from build123d import *

# Parameters (mm, degrees)
CYLINDER001_R     = 1.5
CYLINDER001_DEPTH = 40
CYLINDER_R        = 1.5
CYLINDER_DEPTH    = 40
BOX003_W          = 10
BOX003_H          = 40
BOX003_DEPTH      = 25
BOX002_W          = 5
BOX002_H          = 35
BOX002_DEPTH      = 35
BOX001_W          = 10
BOX001_H          = 40
BOX001_DEPTH      = 25
BOX_W             = 35
BOX_H             = 40
BOX_DEPTH         = 35
FILLET_R          = 10


with BuildPart() as cylinder001:
    # Cylinder001 → Cylinder001 (new body)
    with BuildSketch(Plane(origin=(27.5, 20, 0), x_dir=(1, 0, 0), z_dir=(0, 0, 1))):
        Circle(CYLINDER001_R)
    extrude(amount=CYLINDER001_DEPTH)


with BuildPart() as cylinder:
    # Cylinder → Cylinder (new body)
    with BuildSketch(Plane(origin=(12.5, 20, 0), x_dir=(1, 0, 0), z_dir=(0, 0, 1))):
        Circle(CYLINDER_R)
    extrude(amount=CYLINDER_DEPTH)


with BuildPart() as cube003:
    # Box003 → Box003 (new body)
    with BuildSketch(Plane(origin=(25, 0, 10), x_dir=(1, 0, 0), z_dir=(0, 0, 1))):
        with Locations((5, 20)):
            Rectangle(BOX003_W, BOX003_H)
    extrude(amount=BOX003_DEPTH)


with BuildPart() as cube002:
    # Box002 → Box002 (new body)
    with BuildSketch(Plane(origin=(15, 0, 5), x_dir=(1, 0, 0), z_dir=(0, 0, 1))):
        with Locations((2.5, 17.5)):
            Rectangle(BOX002_W, BOX002_H)
    extrude(amount=BOX002_DEPTH)


with BuildPart() as cube001:
    # Box001 → Box001 (new body)
    with BuildSketch(Plane.XY.offset(10)):
        with Locations((5, 20)):
            Rectangle(BOX001_W, BOX001_H)
    extrude(amount=BOX001_DEPTH)


with BuildPart() as cut004:
    # Box → Box (new body)
    with BuildSketch(Plane.XY):
        with Locations((17.5, 20)):
            Rectangle(BOX_W, BOX_H)
    extrude(amount=BOX_DEPTH)

    # Fillet
    fillet_edges = [cut004.edges().sort_by_distance(p)[0] for p in [
        (0, 0, 17.5),
        (0, 40, 17.5),
        (35, 0, 17.5),
        (35, 40, 17.5),
        (17.5, 0, 35),
        (17.5, 40, 35),
    ]]
    fillet(fillet_edges, radius=FILLET_R)

    # Cut: cut Cube001
    add(cube001.part, mode=Mode.SUBTRACT)

    # Cut001: cut Cube002
    add(cube002.part, mode=Mode.SUBTRACT)

    # Cut002: cut Cube003
    add(cube003.part, mode=Mode.SUBTRACT)

    # Cut003: cut Cylinder
    add(cylinder.part, mode=Mode.SUBTRACT)

    # Cut004: cut Cylinder001
    add(cylinder001.part, mode=Mode.SUBTRACT)


solid = cut004.part
Could you check a few things on this model? Use its own coordinates, in mm. A direction names the side the tool comes from. Give positions to 0.01 mm unless a question says otherwise; leave off trailing zeros. Order: outer loops, then holes, each group sorted by start corner. A loop starts at its lowest first (then second) coordinate and runs counter-clockwise, first axis right, second up. Notation, with made-up numbers: (78, 15.5) - (128, 15.5) arc R16 ccw to (128, 45.5) - close; hole circle Ø7 at (3.25, -26.75). An arc over 180 degrees is marked (long way). One line per item, written item: value. Start each with the question number.
1. For P1, Ø8, axis at x = 5.5, y = 27.5, coming from the +Z side; P2, Ø1.5, axis at y = 13.5, z = 15, coming from the +X side; P3, Ø1.5, axis at x = 17.5, y = 17.5, coming from the +Z side, each with a flat end and sliding along its axis, tell me the tip position at first contact or that it passes through.
2. Imagine slicing it at B-B on z = 20. List the corners of the cut face in (x, y) for me, plus the area to 3 significant figures.
3. If I drill on probe 1 along X at (y, z) = (20, 7); probe 2 along X at (y, z) = (20, 12.5); probe 3 along X at (y, z) = (17.5, 17.5), over which ranges is the centre line in solid material (lowest first)?
4. Imagine slicing it at A-A on x = 12.5. List the corners of the cut face in (y, z) for me.
5. For faces 1 (the face through (25, 20, 22)), 2 (the face through (20, 17, 20)), 3 (the face through (35, 20, 5)), which set-ups out of +Z, -Z, +X, -X, +Y, -Y let a thin tool reach every point of the face, with its end or its side?
6. Imagine slicing it at C-C on y = 20. List the corners of the cut face in (x, z) for me, plus the area to 3 significant figures.
7. Imagine slicing it at D-D on z = 6. List the corners of the cut face in (x, y) for me, plus the area to 3 significant figures.
8. Thinking about a two-plate mould opening in X: for faces 4 (the face through (10, 20, 22)), 5 (the face through (10.8, 20.1, 35)), 6 (the face through (17, 35, 19)), which applies, +X half, -X half, draft (parallel to the pull), parting line (faces both ways), or undercut?
Values:
1. P1: z = 10
1. P2: x = 25
1. P3: z = 5
2. outline: (10, 0) - (15, 0) - (15, 35) - (20, 35) - (20, 0) - (25, 0) - (25, 40) - (10, 40) - close; hole circle Ø3 at (12.5, 20)
2. area: 418 mm²
3. probe 1: 0 to 11, 14 to 15, 20 to 26, 29 to 35
3. probe 2: 10 to 11, 14 to 15, 20 to 25
3. probe 3: 10 to 15, 20 to 25
4. outline: (0, 0) - (18.5, 0) - (18.5, 35) - (10, 35) arc R10 ccw to (0, 25) - close; (21.5, 0) - (40, 0) - (40, 25) arc R10 ccw to (30, 35) - (21.5, 35) - close
5. face 1: +Z, +X, +Y, -Y
5. face 2: +Z, -Y
5. face 3: +Z, -Z, +X, +Y, -Y
6. outline: (0, 0) - (11, 0) - (11, 35) - (10, 35) - (10, 10) - (0, 10) - close; (14, 0) - (26, 0) - (26, 10) - (25, 10) - (25, 35) - (20, 35) - (20, 5) - (15, 5) - (15, 35) - (14, 35) - close; (29, 0) - (35, 0) - (35, 10) - (29, 10) - close
6. area: 440 mm²
7. outline: (0, 10) arc R10 ccw to (10, 0) - (15, 0) - (15, 35) - (20, 35) - (20, 0) - (25, 0) arc R10 ccw to (35, 10) - (35, 30) arc R10 ccw to (25, 40) - (10, 40) arc R10 ccw to (0, 30) - close; hole circle Ø3 at (12.5, 20); hole circle Ø3 at (27.5, 20)
7. area: 1,130 mm²
8. face 4: -X half
8. face 5: draft
8. face 6: undercut
